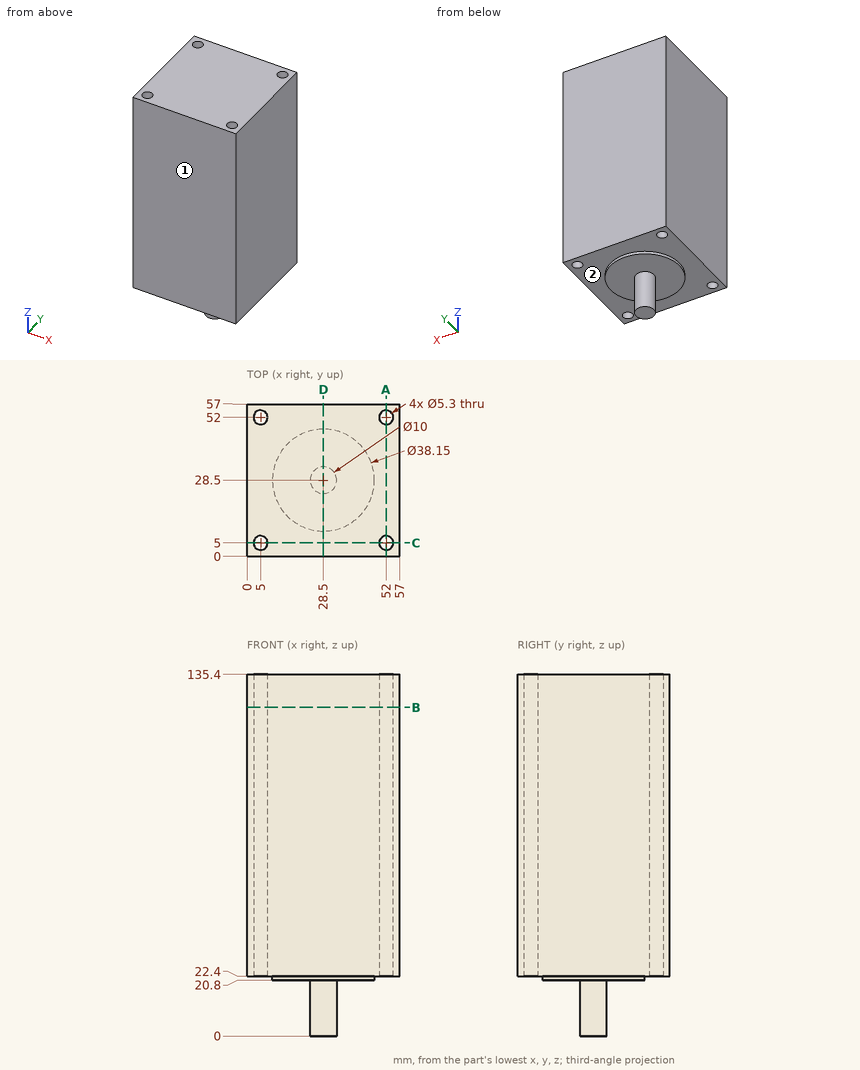
Check sheet for the drawn part. Datum: minimum x, y, z corner. Units: mm. A direction names the side the tool comes from. Give positions to 0.01 mm unless a question says otherwise; leave off trailing zeros. Write each loop counter-clockwise with the first axis right and the second up, starting at its lowest first coordinate (ties: lowest second). Pieces come first, ordered by that corner, then holes.
(1) Material ranges on line 1 (Y direction, x = 5, z = 79.5); line 2 (Y direction, x = 6, z = 99.5); line 3 (Z direction, x = 18, y = 36.5), recorded low to high.
(2) Cross-section at D-D (x = 28.5). Enter the section's corners in (y, z) (3 decimals).
(3) Access from +Z, -Z, +X, -X, +Y, -Y to the whole of each face (thin tool, end or side, straight path). Record for the marked faces 1 and 2.
(4) Cross-section at B-B (z = 123). Enter the section's corners in (x, y), plus the area to 3 significant figures.
(5) Gauge pin test, flat ends, axial feed: pin 1 (6 mm diameter, centred on x = 52, y = 5, fed in from -Z); pin 2 (4 mm diameter, centred on x = 28, y = 21, fed in from -Z). Record the tip position at first contact, or that the pin passes through.
(6) Cross-section at A-A (x = 52). Enter the section's corners in (y, z), plus the area to 3 significant figures.
Worked out:
1. line 1: y = 0 to 2.35, 7.65 to 49.35, 54.65 to 57
1. line 2: y = 0 to 2.55, 7.45 to 49.55, 54.45 to 57
1. line 3: z = 20.8 to 135.4
2. outline: (0, 22.4) - (9.425, 22.4) - (9.425, 20.8) - (23.5, 20.8) - (23.5, 0) - (33.5, 0) - (33.5, 20.8) - (47.575, 20.8) - (47.575, 22.4) - (57, 22.4) - (57, 135.4) - (0, 135.4) - close
3. face 1: +Z, -Z, +X, -X, -Y
3. face 2: -Z
4. outline: (0, 0) - (57, 0) - (57, 57) - (0, 57) - close; hole circle Ø5.3 at (5, 5); hole circle Ø5.3 at (5, 52); hole circle Ø5.3 at (52, 5); hole circle Ø5.3 at (52, 52)
4. area: 3,160 mm2
5. pin 1: stops at z = 22.4
5. pin 2: stops at z = 20.8
6. outline: (0, 22.4) - (2.35, 22.4) - (2.35, 135.4) - (0, 135.4) - close; (7.65, 22.4) - (49.35, 22.4) - (49.35, 135.4) - (7.65, 135.4) - close; (54.65, 22.4) - (57, 22.4) - (57, 135.4) - (54.65, 135.4) - close
6. area: 5,240 mm2
